Source: CAD feature listing. Evaluate the final solid. Frame: model axes, mm. Face numbers are marked on the shaded views. A direction names the side the tool comes from. Round coordinates to 2 decimals unless told otherwise and drop trailing zeros. Loops run counter-clockwise (first coordinate to the right, second up) from the corner with the lowest first, then second, coordinate; pieces in that order, holes last.
(1) Section D-D, the plane x = -13. Return the cut outline in (y, z), plus the area to 3 significant figures.
(2) Section B-B, the plane x = 6.5. Return the cut outline in (y, z), plus the area to 3 significant figures.
(3) Set-up query: the marked faces 5, 6 and 7. Return all of +Z, -Z, +X, -X, +Y, -Y with unobstructed straight access to the full face (end or side cutting, diameter ignored); none if empty.
(4) Section C-C, the plane x = 16. Return the cut outline in (y, z).
(5) Section A-A, the plane y = 44. Return the cut outline in (x, z), plus the area to 3 significant figures.
(6) Mould query, pull axis X, two halves, no side actions, for the marked faces 1, 2, 3 and 4. Classes: pulls with the +X half, pulls with the -X half, needs draft (parallel to the pull), parting line crosses it, or undercut.
(7) First-contact query: pin 1 Ø8 at (x, y) = (-17.5, 12.5) entering from -Z; pin 2 Ø6 at (y, z) = (17.5, -35) entering from +X; pin 3 Ø3 at (x, y) = (11.5, 31.5) entering from -Z. Flat tips, straight axial feed; report the tip coordinate or a pass-through.
(8) Material intervals for probe 1 along Y at (x, z) = (-11, -28); probe 2 along Y at (x, z) = (14, -27); probe 3 along X at (y, z) = (28, -2), sorted ascending.
```python
from build123d import *

# Parameters (mm, degrees)
BOSS_EXTRUDE1_DEPTH = 20
BOSS_EXTRUDE2_DEPTH = 10
CUT_EXTRUDE1_DEPTH  = 71.178344238


with BuildPart() as part:
    # Sketch1 → Boss-Extrude1 (new, symmetric)
    with BuildSketch(Plane(origin=(0, 0, 0), x_dir=(0, 0, -1), z_dir=(1, 0, 0))):
        with BuildLine():
            ThreePointArc((20, 0), (14.142135624, 14.142135624), (0, 20))
            Line((0, 20), (0, 50))
            Line((0, 50), (10, 50))
            Line((10, 50), (30, 25))
            Line((30, 25), (30, 0))
            Line((30, 0), (20, 0))
        make_face()
    extrude(amount=BOSS_EXTRUDE1_DEPTH, both=True)

    # Sketch1_3 → Boss-Extrude2 (add, symmetric)
    with BuildSketch(Plane(origin=(0, 0, 0), x_dir=(0, 0, -1), z_dir=(1, 0, 0))):
        Polygon((30, 0), (45, 0), (30, 25), align=None)
    extrude(amount=BOSS_EXTRUDE2_DEPTH, both=True)

    # Sketch2 → Cut-Extrude1 (cut, through all)
    with BuildSketch(Plane.XY):
        Polygon((15, 25), (5, 50), (-5, 50), (-15, 25), align=None)
    extrude(amount=-CUT_EXTRUDE1_DEPTH, mode=Mode.SUBTRACT)


solid = part.part
```
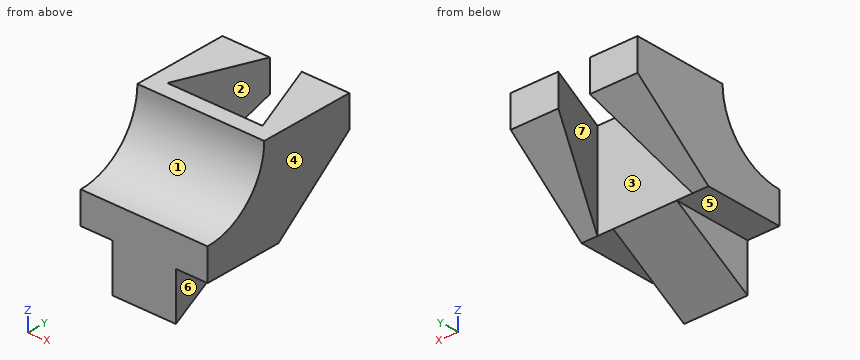
Output values:
1. outline: (0, -30) - (25, -30) - (25, 0) - (20, 0) arc R20 cw to (0, -20) - close; (30, -26) - (50, -10) - (50, 0) - (30, 0) - close
1. area: 796 mm2
2. outline: (0, -45) - (25, -30) - (25, 0) - (20, 0) arc R20 cw to (0, -20) - close; (46.25, -13) - (50, -10) - (50, 0) - (46.25, 0) - close
2. area: 666 mm2
3. face 5: -Z, -X, +Y, -Y
3. face 6: -Z, +X, +Y, -Y
3. face 7: +Z, -Z
4. outline: (0, -30) - (25, -30) - (50, -10) - (50, 0) - (20, 0) arc R20 cw to (0, -20) - close
5. outline: (-20, -14.8) - (-7.4, -14.8) - (-7.4, 0) - (-20, 0) - close; (7.4, -14.8) - (20, -14.8) - (20, 0) - (7.4, 0) - close
5. area: 373 mm2
6. face 1: needs draft
6. face 2: undercut
6. face 3: undercut
6. face 4: pulls with the +X half
7. pin 1: stops at z = -30
7. pin 2: stops at x = 10
7. pin 3: stops at z = -25.48
8. probe 1: y = 0 to 25
8. probe 2: y = 0 to 25, 27.5 to 28.75
8. probe 3: x = -20 to -13.8, 13.8 to 20
